Can you work these out from the model? Positions are in its coordinate system, mm. A direction names the side the tool comes from. Give positions to 0.01 mm unless a question says otherwise; leave off trailing zeros. Loops run counter-clockwise (first coordinate to the right, second up) from the corner with the lowest first, then second, coordinate; pieces in that order, holes last. Notation, with made-up numbers: (63.25, -0.5) - (67.25, -0.5) arc R16 ccw to (67.25, 26.5) - close; hole circle Ø4 at (26.25, -11). An arc over 180 degrees is marked (long way). Answer as a JSON object with one key per item and string values.
```python
from build123d import *

# Parameters (mm, degrees)
F0_W      = 63.5
F0_H      = 38.1
F1_DEPTH  = 25.4
F3_DEPTH  = 38.1
F4_W      = 44.45
F4_H      = 12.7
F5_DEPTH  = 19.05
F6_W      = 6.35
F6_H      = 38.1
F7_DEPTH  = 19.05
F8_W      = 6.35
F8_H      = 38.1
F9_DEPTH  = 19.05
F10_R     = 5.08
F11_W     = 7.62
F11_H     = 19.05
F12_DEPTH = 19.05
F13_R     = 5.08
F14_W     = 7.62
F14_H     = 19.05
F15_DEPTH = 19.05
F16_R     = 5.08


with BuildPart() as f1:
    # F0 (on Front) → F1 (new body)
    with BuildSketch(Plane.XZ):
        Rectangle(F0_W, F0_H)
    extrude(amount=F1_DEPTH)

    # F2 (on face) → F3 (cut)
    with BuildSketch(Plane.XZ.offset(25.4)):
        with BuildLine():
            Line((12.7, 19.05), (-12.7, 19.05))
            ThreePointArc((-12.7, 19.05), (0, 6.35), (12.7, 19.05))
        make_face()
    extrude(amount=-F3_DEPTH, mode=Mode.SUBTRACT)

    # F4 (on face) → F5 (cut)
    with BuildSketch(Plane.XZ.offset(25.4)):
        with Locations((0, -12.7)):
            Rectangle(F4_W, F4_H)
    extrude(amount=-F5_DEPTH, mode=Mode.SUBTRACT)

    # F6 (on face) → F7 (cut)
    with BuildSketch(Plane.XZ.offset(25.4)):
        with Locations((-28.575, 0)):
            Rectangle(F6_W, F6_H)
    extrude(amount=-F7_DEPTH, mode=Mode.SUBTRACT)

    # F8 (on face) → F9 (cut)
    with BuildSketch(Plane.XZ.offset(25.4)):
        with Locations((28.575, 0)):
            Rectangle(F8_W, F8_H)
    extrude(amount=-F9_DEPTH, mode=Mode.SUBTRACT)

    # F10
    f10_edges = [f1.edges().sort_by_distance(p)[0] for p in [
        (31.75, -3.175, 19.05),
        (-31.75, -3.175, 19.05),
    ]]
    fillet(f10_edges, radius=F10_R)

    # F11 (on face) → F12 (cut)
    with BuildSketch(Plane.XZ.offset(25.4)):
        with Locations((-21.59, 9.525)):
            Rectangle(F11_W, F11_H)
    extrude(amount=-F12_DEPTH, mode=Mode.SUBTRACT)

    # F13
    f13_edges = [f1.edges().sort_by_distance(p)[0] for p in [
        (-17.78, -15.875, 0),
    ]]
    fillet(f13_edges, radius=F13_R)

    # F14 (on face) → F15 (cut)
    with BuildSketch(Plane.XZ.offset(25.4)):
        with Locations((21.59, 9.525)):
            Rectangle(F14_W, F14_H)
    extrude(amount=-F15_DEPTH, mode=Mode.SUBTRACT)

    # F16
    f16_edges = [f1.edges().sort_by_distance(p)[0] for p in [
        (17.78, -15.875, 0),
    ]]
    fillet(f16_edges, radius=F16_R)


solid = f1.part
```
1) Which directions (+Z, -Z, +X, -X, +Y, -Y) give clear straight access to the entire face, cutting with the end or side of a thin tool? Please do faces 5 (the flat face through (-25.4, -16, -10)), 6 (the flat face through (17.78, -16, 12)), 7 (the cylindrical face through (-19.229, -15.742, 1.528)), 8 (the cylindrical face through (30.222, -3.219, 17.601)), 9 (the flat face through (0, -6.35, -13)).
Check sheet entries:
{"face 5": "+Z, -Z, -X, -Y", "face 6": "+Z, +X, -Y", "face 7": "+Z, -X, -Y", "face 8": "+Z, +X, +Y, -Y", "face 9": "-Z, -Y"}
2) I'm going to push flat-ended pins straight in: P1, Ø8, axis at x = 25, z = 5.5, coming from the -Y side; P2, Ø15, axis at x = -1, y = -20.5, coming from the -Z side; P3, Ø15, axis at y = -17, z = -5, coming from the -X side; P4, Ø12, axis at x = -23.5, z = 10.5, coming from the -Y side. Where does each tip first touch, or does it pass through?
Check sheet entries:
{"P1": "y = -6.35", "P2": "z = -6.35", "P3": "x = -25.4", "P4": "y = -25.4"}
3) Imagine slicing it at C-C on y = -9.75. Write out the boundary of the cut face in (x, z) (3 decimals), and give its area (3 significant figures).
Check sheet entries:
{"outline": "(-25.4, -19.05) - (-22.225, -19.05) - (-22.225, -6.35) - (22.225, -6.35) - (22.225, -19.05) - (25.4, -19.05) - (25.4, 0) - (22.86, 0) arc R5.08 cw to (17.78, 5.08) - (17.78, 19.05) - (12.7, 19.05) arc R12.7 cw to (-12.7, 19.05) - (-17.78, 19.05) - (-17.78, 5.08) arc R5.08 cw to (-22.86, 0) - (-25.4, 0) - close", "area": "838 mm2"}
4) I need wall thicknesses on L1, parallel to X at y = -22.5, z = -9 (3 decimals); L2, parallel to X at y = -8.5, z = -5.5; L3, parallel to Z at x = 11, y = -6. Which ranges of each line are inside material? Lowest first, please.
Check sheet entries:
{"L1": "-25.4 to -22.225, 22.225 to 25.4", "L2": "-25.4 to 25.4", "L3": "-19.05 to 12.7"}
5) Imagine slicing it at A-A on z = 8. Write out the boundary of the cut face in (x, y), and give its area (3 significant figures).
Check sheet entries:
{"outline": "(-31.75, -6.35) - (-17.78, -6.35) - (-17.78, -25.4) - (-6.26, -25.4) - (-6.26, 0) - (-31.75, 0) - close; (6.26, -25.4) - (17.78, -25.4) - (17.78, -6.35) - (31.75, -6.35) - (31.75, 0) - (6.26, 0) - close", "area": "763 mm2"}
6) Imagine slicing it at B-B on z = -7.5. Write out the boundary of the cut face in (x, y) (3 decimals).
Check sheet entries:
{"outline": "(-31.75, -6.35) - (-25.4, -6.35) - (-25.4, -25.4) - (-22.225, -25.4) - (-22.225, -6.35) - (22.225, -6.35) - (22.225, -25.4) - (25.4, -25.4) - (25.4, -6.35) - (31.75, -6.35) - (31.75, 0) - (-31.75, 0) - close"}
7) Imagine slicing it at D-D on x = -20. Write out the boundary of the cut face in (y, z), and give its area (3 significant figures).
Check sheet entries:
{"outline": "(-25.4, -6.35) - (-6.35, -6.35) - (-6.35, -19.05) - (0, -19.05) - (0, 19.05) - (-6.35, 19.05) - (-6.35, 0.88) - (-25.4, 0.88) - close", "area": "380 mm2"}
8) If we mould it in two halves opening along X, with no side actions, what happens to faces 1 (the flat face through (25.4, -16, -10)), 2 (the cylindrical face through (-0.279, -12.878, 6.353)), 3 (the flat face through (0, -16, -6.35)), 4 (the flat face through (16, -10, 19.05))? For each: released by +X, released by -X, zero draft, split by the parting line, or undercut.
Check sheet entries:
{"face 1": "released by +X", "face 2": "undercut", "face 3": "undercut", "face 4": "zero draft"}
